```python
from build123d import *

# Parameters (mm, degrees)
F1_DEPTH    = 3.81
F2_T1_DEPTH = 8.770689479
F2_T3_DEPTH = 9.6298711326
F3_R        = 3.81
F4_R        = 5.08
F5_R        = 1.27
F6_R        = 1.27


# Not quite as in the source:
# - a fillet or chamfer that OpenCascade refuses, or shapes differently, is made with other operations: its cross-section is extruded or revolved along the edge and cut away or added


with BuildPart() as f1:
    # F0 (on Front) → F1 (new body)
    with BuildSketch(Plane.XZ):
        Polygon((0, 5.842), (0, 0), (24.0501028134, 0), (29.035013032, 8.6341177699), (54.7257371953, 1.27), (54.7257371953, 0), (69.088, 0), (69.088, 5.08), (24.657370278, 17.8158181024), (23.9974589203, 16.6728181024), (24.657370278, 16.2918181024), (19.577370278, 7.493), (12.4283305697, 11.6205), (14.9683305697, 16.0199090512), (8.1492465403, 19.9569090512), align=None)
    extrude(amount=F1_DEPTH)

    # F2: fillet of radius 1.27 on 2 edges, made by hand

    # F2_s2 → F2_t1 (cut)
    with BuildSketch(Plane.XZ.offset(-2.4803447395)):
        with BuildLine():
            ThreePointArc((25.6110997962, 17.5424362994), (24.7853486084, 17.4991029103), (24.16130133, 16.9566014806))
            Line((24.16130133, 16.9566014806), (24.657370278, 17.8158181024))
            Line((24.657370278, 17.8158181024), (25.6110997962, 17.5424362994))
        make_face()
    extrude(amount=F2_T1_DEPTH, mode=Mode.SUBTRACT)

    # F2_s4 → F2_t3 (cut)
    with BuildSketch(Plane.XZ.offset(-2.9099355663)):
        with BuildLine():
            ThreePointArc((24.5794460335, 17.680849352), (24.4112920489, 16.9747145746), (24.657370278, 16.2918181024))
            Line((24.657370278, 16.2918181024), (23.9974589203, 16.6728181024))
            Line((23.9974589203, 16.6728181024), (24.5794460335, 17.680849352))
        make_face()
    extrude(amount=F2_T3_DEPTH, mode=Mode.SUBTRACT)

    # F3
    f3_edges = [f1.edges().sort_by_distance(p)[0] for p in [
        (8.149247, -1.905, 19.956909),
    ]]
    fillet(f3_edges, radius=F3_R)

    # F4
    f4_edges = [f1.edges().sort_by_distance(p)[0] for p in [
        (69.088, -1.905, 5.08),
    ]]
    fillet(f4_edges, radius=F4_R)

    # F5
    f5_edges = [f1.edges().sort_by_distance(p)[0] for p in [
        (29.035013, -1.905, 8.634118),
        (24.050103, -1.905, 0),
        (54.725737, -1.905, 1.27),
    ]]
    fillet(f5_edges, radius=F5_R)

    # F6
    f6_edges = [f1.edges().sort_by_distance(p)[0] for p in [
        (54.725737, -1.905, 0),
    ]]
    fillet(f6_edges, radius=F6_R)


solid = f1.part
```
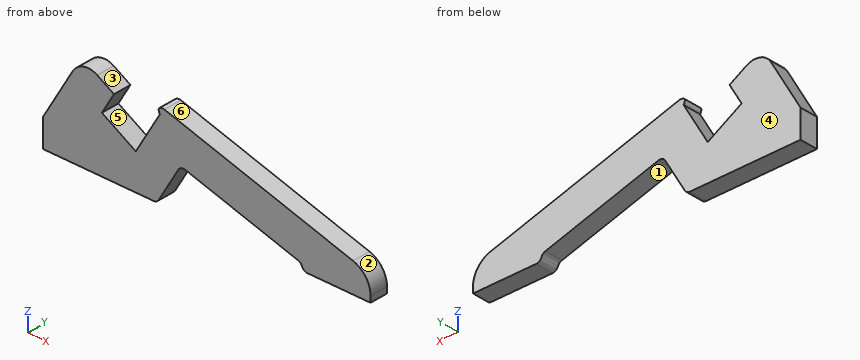
Input: part model. Units: mm. Frame: model coordinates. Face numbers are marked on the shaded views. A direction names the side the tool comes from. Give positions to 0.01 mm unless a question says otherwise; leave off trailing zeros. Order: outer loops, then holes, each group sorted by start corner. A loop starts at its lowest first (then second) coordinate and runs counter-clockwise, first axis right, second up. Notation, with made-up numbers: (20.25, 67) - (24.25, 67) arc R19 cw to (24.25, 82) - close; hole circle Ø10 at (57, 24.25). An arc over 180 degrees is marked (long way). Use a Markdown table: item, result.
(1) Pin query (flat end, axial travel): pin 1 (1 mm diameter, centred on x = 57, z = 10.5, fed in from +Y). Return the tip coordinate at first contact, or that it passes through.
Computed values:
| item | result |
|---|---|
| pin 1 | passes through |
(2) Line query: line 1 (Z direction, x = 36, y = -1.7); line 2 (Z direction, x = 55, y = -1.25). Output: solid intervals per line, ascending. Write a range as from..to.
Computed values:
| item | result |
|---|---|
| line 1 | z = 6.64..14.56 |
| line 2 | z = 0.29..9.12 |
(3) Section query C-C (x = 62). Output: boundary loops of the cut face in (y, z), then the cut area to 3 significant figures.
Computed values:
| item | result |
|---|---|
| outline | (-3.81, 0) - (0, 0) - (0, 7.11) - (-3.81, 7.11) - close |
| area | 27.1 mm2 |
(4) Draft query along X for the marked faces 4, 5 and 6. Return one class per face: released by +X, released by -X, zero draft, split by the parting line, or undercut.
Computed values:
| item | result |
|---|---|
| face 4 | zero draft |
| face 5 | undercut |
| face 6 | released by +X |
(5) Access query for the marked faces 1, 2 and 3. Directions: +Z, -Z, +X, -X, +Y, -Y. A direction counts if a zero-diameter tool reaches every point of the face in a straight line with its end or side. Return the directions, or none.
Computed values:
| item | result |
|---|---|
| face 1 | -Z, +Y, -Y |
| face 2 | +Z, +X, +Y, -Y |
| face 3 | +Z, +Y, -Y |
(6) Section query B-B (z = 3.25). Output: boundary loops of the cut face in (x, y), then the cut area to 3 significant figures.
Computed values:
| item | result |
|---|---|
| outline | (0, -3.81) - (25.93, -3.81) - (25.93, 0) - (0, 0) - close; (47.82, -3.81) - (68.68, -3.81) - (68.68, 0) - (47.82, 0) - close |
| area | 178 mm2 |
(7) Section query D-D (x = 38.5). Output: boundary loops of the cut face in (y, z), then the cut area to 3 significant figures.
Computed values:
| item | result |
|---|---|
| outline | (-3.81, 5.92) - (0, 5.92) - (0, 13.85) - (-3.81, 13.85) - close |
| area | 30.2 mm2 |
(8) Section query A-A (z = 12.5). Output: boundary loops of the cut face in (x, y), then the cut area to 3 significant figures.
Computed values:
| item | result |
|---|---|
| outline | (3.84, -3.81) - (12.94, -3.81) - (12.94, 0) - (3.84, 0) - close; (22.47, -3.81) - (43.2, -3.81) - (43.2, 0) - (22.47, 0) - close |
| area | 114 mm2 |
